Check sheet for the modelled part. Datum: model origin and axes. Units: mm. Face numbers are marked on the shaded views. A direction names the side the tool comes from. Give positions to 0.01 mm unless a question says otherwise; leave off trailing zeros. Loops run counter-clockwise (first coordinate to the right, second up) from the corner with the lowest first, then second, coordinate; pieces in that order, holes last. Notation, with made-up numbers: (-20.75, 78) - (38.25, 78) arc R24 ccw to (38.25, 97) - close; hole circle Ø1 at (-4, -31). An arc over 180 degrees is marked (long way). Answer in a Markdown table with one row per item. Add a question column.
(1) Sectioned sample at C-C on x = -15.5. Enter the section's corners in (y, z).
(2) Sectioned sample at B-B on z = -15.5. Enter the section's corners in (x, y).
(3) Set-up check for the marked faces 1 and 2: record each of +Z, -Z, +X, -X, +Y, -Y from which the full face is reachable in a straight line by a thin tool's end or side.
(4) Sectioned sample at A-A on x = 0. Enter the section's corners in (y, z).
(5) Thickness scan on L1, parallel to X at y = 36.15, z = -15.5; L2, parallel to Y at x = -11.5, z = -4. Record the ranges inside material, lowest first.
(6) Sectioned sample at D-D on y = 41.5. Enter the section's corners in (x, z).
(7) Go/stop test with flat-tipped pins: P1, Ø2.5, axis at x = 15.5, z = 15.5, coming from the +Y side; P2, Ø2.5, axis at x = 16, z = -15, coming from the +Y side; P3, Ø6, axis at x = 3, z = 8.5, coming from the +Y side. Record where each tip stops, or that it passes through.
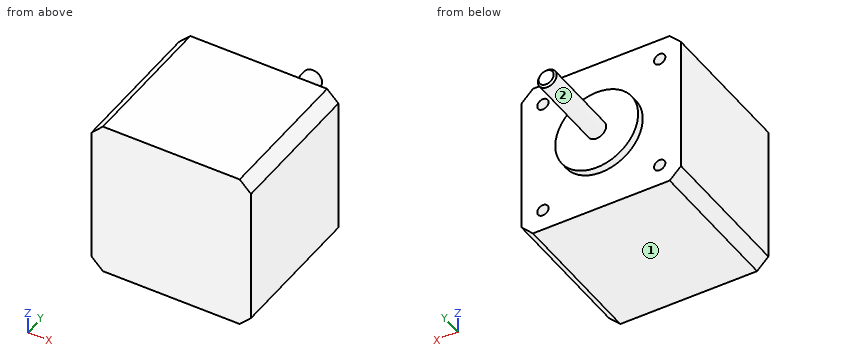
Autodesk Inventor part; units mm, degrees
ref_plane "YZ Plane" through (0, 0, 0) normal (1, 0, 0) x (0, 1, 0)
ref_plane "XZ Plane" through (0, 0, 0) normal (0, 1, 0) x (-1, 0, 0)
ref_plane "XY Plane" through (0, 0, 0) normal (0, 0, 1) x (1, 0, 0)
sketch "Sketch1" plane through (0, 0, 0) normal (0, 1, 0) x (-1, 0, 0)
  line L0 (21.15, 21.15) -> (-21.15, 21.15)
  line L1 (-21.15, 21.15) -> (-21.15, -21.15)
  line L2 (-21.15, -21.15) -> (21.15, -21.15)
  line L3 (21.15, -21.15) -> (21.15, 21.15)
  point P0 (0, 0)
  point P1 (21.15, 0)
  point P2 (0, -21.15)
  dimension "d0" = 42.3
  dimension "d1" = 42.3
extrude "Extrusion1" add sketch "Sketch1" along normal blind 38
chamfer "Chamfer1" distance 3 angle 45 4 edges at (21.15, 19, 21.15) (21.15, 19, -21.15) (-21.15, 19, -21.15) (-21.15, 19, 21.15)
sketch "Sketch2" plane through (0, 38, 0) normal (0, 1, 0) x (1, 0, 0)
  circle A0 centre (0, 0) radius 11
  dimension "d7" = 22
extrude "Extrusion2" add sketch "Sketch2" along normal blind 2
sketch "Sketch3" plane through (0, 40, 0) normal (0, 1, 0) x (1, 0, 0)
  circle A0 centre (0, 0) radius 2.5
  dimension "d10" = 5
extrude "Extrusion3" add sketch "Sketch3" along normal blind 22
chamfer "Chamfer2" distance 0.5 angle 45 1 edges at (-2.5, 62, 0)
sketch "Sketch4" plane through (0, 38, 0) normal (0, 1, 0) x (1, 0, 0)
  circle A0 centre (15.5, 15.5) radius 1.5
  circle A1 centre (15.5, -15.5) radius 1.5
  circle A2 centre (-15.5, -15.5) radius 1.5
  circle A3 centre (-15.5, 15.5) radius 1.5
  line L0 (21.15, -18.15) -> (21.15, 18.15)
  line L1 (18.15, 21.15) -> (-18.15, 21.15)
  line L2 (-21.15, 18.15) -> (-21.15, -18.15)
  line L3 (-18.15, -21.15) -> (18.15, -21.15)
  point P0 (0, 0)
  dimension "d16" = 3
  dimension "d17" = 3
  dimension "d18" = 3
  dimension "d19" = 3
  dimension "d20" = 5.65
  dimension "d21" = 5.65
  dimension "d24" = 5.65
  dimension "d25" = 5.65
extrude "Extrusion4" cut sketch "Sketch4" against normal blind 4
properties part number "Stepper Motor"
Reply:
| question | item | result |
|---|---|---|
| 1 | outline | (0, -21.15) - (38, -21.15) - (38, -17) - (34, -17) - (34, -14) - (38, -14) - (38, 14) - (34, 14) - (34, 17) - (38, 17) - (38, 21.15) - (0, 21.15) - close |
| 2 | outline | (-21.15, 0) - (21.15, 0) - (21.15, 38) - (17, 38) - (17, 34) - (14, 34) - (14, 38) - (-14, 38) - (-14, 34) - (-17, 34) - (-17, 38) - (-21.15, 38) - close |
| 3 | face 1 | -Z, +X, -X, +Y, -Y |
| 3 | face 2 | +Y |
| 4 | outline | (0, -21.15) - (38, -21.15) - (38, -11) - (40, -11) - (40, -2.5) - (61.5, -2.5) - (62, -2) - (62, 2) - (61.5, 2.5) - (40, 2.5) - (40, 11) - (38, 11) - (38, 21.15) - (0, 21.15) - close |
| 5 | L1 | -21.15 to -17, -14 to 14, 17 to 21.15 |
| 5 | L2 | 0 to 38 |
| 6 | outline | circle Ø5 at (0, 0) |
| 7 | P1 | y = 34 |
| 7 | P2 | y = 38 |
| 7 | P3 | y = 40 |
